The listing builds one solid part. Answer for the finished solid, in the listing's coordinates (mm). Face numbers are marked on the shaded views. A direction names the side the tool comes from. Round coordinates to 2 decimals unless told otherwise and drop trailing zeros. Order: outer loops, then holes, each group sorted by start corner. A loop starts at its lowest first (then second) coordinate and runs counter-clockwise, first axis right, second up. Notation, with made-up numbers: (-3.5, -0.5) -> (11.5, -0.5) arc R15 ccw to (11.5, 14.5) -> close; hole circle Ø8 at (52.5, -3.5). An arc over 180 degrees is marked (long way). Return JSON: item names as keys, results as strings. Group by question number.
(1) Which of the six approach directions +Z, -Z, +X, -X, +Y, -Y give full straight-line access (tool end or side, diameter ignored) to the marked faces 1 and 2?
(2) Each of these flat-tipped pins is pushed along its axis until it touches: pin 1 (5 mm diameter, centred on y = -2, z = -0.5, fed in from +X); pin 2 (2 mm diameter, centred on x = 17.5, y = 16, fed in from -Z); pin 3 (10 mm diameter, centred on x = -0.5, y = -0.5, fed in from +Z). Where does it stop, or does it pass through?
(3) The part is cut by section D-D (x = -31). Determine the outline of the cut face in (y, z), plus the area to 3 significant figures.
(4) Determine the mould class of the marked faces 3, 4 and 5 for opening direction Y: +Y half, -Y half, draft (parallel to the pull), parting line (faces both ways), or undercut.
(5) The part is cut by section B-B (z = 17.5). Determine the outline of the cut face in (x, y).
(6) The part is cut by section A-A (x = 0). Determine the outline of the cut face in (y, z).
(7) Consider line 1 (Y direction, x = 1.5, z = 12.5); line 2 (Z direction, x = -6, y = -5); line 3 (X direction, y = 12, z = -0.5). Determine where each line is inside the solid, lowest interval first. Write a range as [from, to].
(8) The part is cut by section C-C (z = 12). Count the separate pieces of the cut face and the enclosed holes in it, plus the area to 3 significant figures.
from build123d import *

# Parameters (mm, degrees)
SKETCH_1_W                       = 20
SKETCH_1_H                       = 34
SM_BASE_FLANGE_1_DEPTH           = 2
SM_EDGE_FLANGE_1_STRIP_W         = 13.4732
SM_EDGE_FLANGE_1_STRIP_H         = 2
SM_EDGE_FLANGE_1_STRIP_CUT_DEPTH = 20
SM_EDGE_FLANGE_1_DEPTH           = 20
SM_EDGE_FLANGE_1_FLAT_DEPTH      = 2
SKETCH_9_R                       = 2.75
CUT_EXTRUDE_1_DEPTH              = 55.693859429


# Sheet-metal steps are written as plain solids
with BuildPart() as part:
    # Sketch 1 → 基体-法兰1 (new body)
    with BuildSketch(Plane.XY):
        Rectangle(SKETCH_1_W, SKETCH_1_H)
    extrude(amount=-SM_BASE_FLANGE_1_DEPTH)

    # 边线-法兰1 strip (across the edge) → 边线-法兰1 strip cut (cut)
    with BuildSketch(Plane(origin=(10, 17, 0), x_dir=(0, -1, 0), z_dir=(-1, 0, 0))):
        with Locations((-2, -1)):
            Rectangle(SM_EDGE_FLANGE_1_STRIP_W, SM_EDGE_FLANGE_1_STRIP_H)
    sm_edge_flange_1_strip_cut = extrude(amount=SM_EDGE_FLANGE_1_STRIP_CUT_DEPTH, mode=Mode.SUBTRACT)

    # 边线-法兰1 bend section (across the edge) → 边线-法兰1 (add)
    with BuildSketch(Plane(origin=(10, 17, 0), x_dir=(0, -1, 0), z_dir=(-1, 0, 0))):
        with BuildLine():
            Line((0, 2.7366), (2, 2.7366))
            ThreePointArc((2, 2.7366), (2.801531583, 0.801531583), (4.7366, 0))
            Line((4.7366, 0), (4.7366, -2))
            ThreePointArc((4.7366, -2), (1.38731802, -0.61268198), (0, 2.7366))
        make_face()
    sm_edge_flange_1 = extrude(amount=SM_EDGE_FLANGE_1_DEPTH)

    # 边线-法兰1 profile (on flange) → 边线-法兰1 flat (add)
    with BuildSketch(Plane.XZ.offset(-17)):
        with BuildLine():
            ThreePointArc((23.293714059, 23.066675634), (0, 20), (-23.293714059, 23.066675634))
            ThreePointArc((-23.293714059, 23.066675634), (-35.541162773, 15.995607822), (-28.470094961, 3.748159108))
            Line((-28.470094961, 3.748159108), (-24.025119684, 2.7366))
            Line((-24.025119684, 2.7366), (24.025119684, 2.7366))
            Line((24.025119684, 2.7366), (28.470094961, 3.748159108))
            ThreePointArc((28.470094961, 3.748159108), (35.541162773, 15.995607822), (23.293714059, 23.066675634))
        make_face()
    sm_edge_flange_1_flat = extrude(amount=SM_EDGE_FLANGE_1_FLAT_DEPTH)

    # 镜向1: 边线-法兰1 strip cut, 边线-法兰1, 边线-法兰1 flat across plane
    add(sm_edge_flange_1_strip_cut.mirror(Plane.ZX), mode=Mode.SUBTRACT)
    add(sm_edge_flange_1.mirror(Plane.ZX))
    add(sm_edge_flange_1_flat.mirror(Plane.ZX))

    # 草图9 → 切除-拉伸1 (cut, through all)
    with BuildSketch(Plane(origin=(0, 17, 0), x_dir=(1, 0, 0), z_dir=(0, 1, 0))):
        with Locations(Location((0, -10, 0), (0, 0, 270))):
            Circle(SKETCH_9_R)
        with Locations(Location((25.88190451, -13.407417371, 0), (0, 0, 270))):
            Circle(SKETCH_9_R)
        with Locations(Location((-25.88190451, -13.407417371, 0), (0, 0, 270))):
            Circle(SKETCH_9_R)
    extrude(amount=-CUT_EXTRUDE_1_DEPTH, mode=Mode.SUBTRACT)


solid = part.part
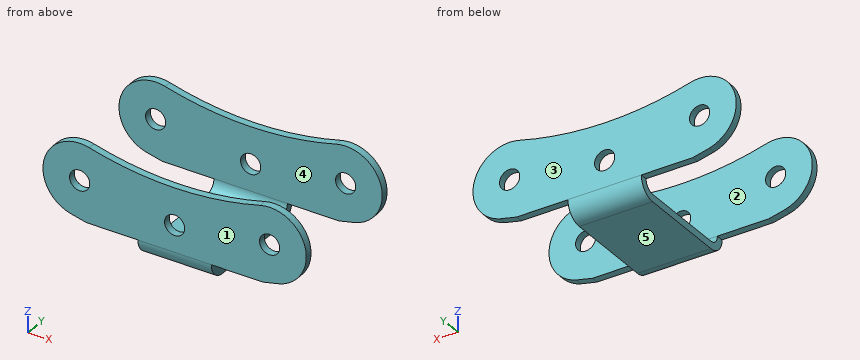
Answer below:
{
 "1": {"face 1": "+Z, -Z, +X, -X, -Y", "face 2": "+Z, +X, -X"},
 "2": {"pin 1": "stops at x = 10", "pin 2": "stops at z = 2.74", "pin 3": "stops at z = 0"},
 "3": {"outline": "(-17, 4.82) -> (-15, 4.82) -> (-15, 22) -> (-17, 22) -> close; (15, 4.82) -> (17, 4.82) -> (17, 22) -> (15, 22) -> close", "area": "68.7 mm²"},
 "4": {"face 3": "+Y half", "face 4": "undercut", "face 5": "draft"},
 "5": {"outline": "(-35.01, -17) -> (35.01, -17) -> (35.01, -15) -> (-35.01, -15) -> close; (-35.01, 15) -> (35.01, 15) -> (35.01, 17) -> (-35.01, 17) -> close"},
 "6": {"outline": "(-17, 2.74) arc R4.74 ccw to (-12.26, -2) -> (12.26, -2) arc R4.74 ccw to (17, 2.74) -> (17, 7.25) -> (15, 7.25) -> (15, 2.74) arc R2.74 cw to (12.26, 0) -> (-12.26, 0) arc R2.74 cw to (-15, 2.74) -> (-15, 7.25) -> (-17, 7.25) -> close; (-17, 12.75) -> (-15, 12.75) -> (-15, 20) -> (-17, 20) -> close; (15, 12.75) -> (17, 12.75) -> (17, 20) -> (15, 20) -> close"},
 "7": {"line 1": "y = [-17, -15], [15, 17]", "line 2": "z = [-2, 0]", "line 3": "x = [-10, 10]"},
 "8": {"separate pieces": "8", "enclosed holes": "0", "area": "233 mm²"}
}
